Check sheet for the modelled part. Datum: model origin and axes. Units: mm. Face numbers are marked on the shaded views. A direction names the side the tool comes from. Coordinates: 2 decimals unless noted, no trailing zeros. Write each loop counter-clockwise with the first axis right and the second up, starting at its lowest first coordinate (ties: lowest second). Pieces come first, ordered by that corner, then holes. Notation, with made-up numbers: M 21.25,10.25 L 28.25,10.25 A13 ccw 28.25,26.25 Z; hole C -4,-12 d4. An arc over 180 degrees is marked long. Answer as CSV lines item,"result". Start each with the question number.
Q1. Thickness scan on line 1 along Y through (x, z) = (-0.5, -3); line 2 along X through (y, z) = (3.5, -1.5). Record the ranges inside material, lowest first. Write a range as from..to.
Q2. Sectioned sample at C-C, the plane x = 0. Record the cut outline in (y, z), then the cut area to 3 significant figures.
Q3. Mould release check, pull along Y, two halves, no side actions. Record for the marked faces 4, 5 and 6: pulls with the +Y half, pulls with the -Y half, needs draft (parallel to the pull), parting line crosses it, or undercut.
Q4. Sectioned sample at A-A, the plane x = -7. Record the cut outline in (y, z).
Q5. Sectioned sample at D-D, the plane z = 0. Record the cut outline in (x, y), then the cut area to 3 significant figures.
Q6. Depth check by flat-ended pin: pin 1 Ø1.1 at (x, y) = (-8.5, 0.5) entering from +Z; pin 2 Ø5 at (x, y) = (2, 10) entering from +Z; pin 3 Ø2 at (x, y) = (-1, 1) entering from +Z. Enter the tip coordinate at first touch or a pass-through.
Q7. Sectioned sample at B-B, the plane z = 5.5. Record the cut outline in (x, y), then the cut area to 3 significant figures.
Q8. Access from +Z, -Z, +X, -X, +Y, -Y to the whole of each face (thin tool, end or side, straight path). Record for the marked faces 1, 2 and 3.
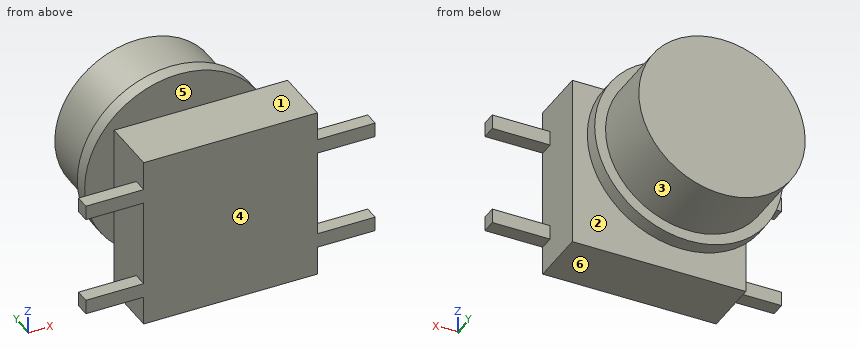
from build123d import *

# Parameters (mm, degrees)
SKETCH1_W               = 12
SKETCH1_H               = 12
BOSS_EXTRUDE1_DEPTH     = 4
SKETCH2_R               = 2.75
BOSS_EXTRUDE2_DEPTH     = 3
SKETCH3_R               = 6.5
BOSS_EXTRUDE3_DEPTH     = 1
BOSS_EXTRUDE4_START     = -1
SKETCH4_R               = 5.75
BOSS_EXTRUDE4_DEPTH     = 5.5
SKETCH5_W               = 1
SKETCH5_H               = 1
BOSS_EXTRUDE5_DEPTH     = 4
MIRROR2_COPY_1_SKETCH_W = 1
MIRROR2_COPY_1_SKETCH_H = 1
MIRROR2_COPY_1_DEPTH    = 4


with BuildPart() as part:
    # Sketch1 → Boss-Extrude1 (new body)
    with BuildSketch(Plane(origin=(0, 0, 0), x_dir=(1, 0, 0), z_dir=(0, 1, 0))):
        Rectangle(SKETCH1_W, SKETCH1_H)
    extrude(amount=BOSS_EXTRUDE1_DEPTH)

    # Sketch2 → Boss-Extrude2 (add)
    with BuildSketch(Plane(origin=(0, 4, 0), x_dir=(1, 0, 0), z_dir=(0, 1, 0))):
        with Locations(Location((0, 0, 0), (0, 0, 270))):
            Circle(SKETCH2_R)
    extrude(amount=BOSS_EXTRUDE2_DEPTH)

    # Sketch3 → Boss-Extrude3 (add)
    with BuildSketch(Plane(origin=(0, 7, 0), x_dir=(1, 0, 0), z_dir=(0, 1, 0))):
        with Locations(Location((0, 0, 0), (0, 0, 270))):
            Circle(SKETCH3_R)
    extrude(amount=BOSS_EXTRUDE3_DEPTH)

    # Sketch4 → Boss-Extrude4 (add)
    with BuildSketch(Plane(origin=(0, 8, 0), x_dir=(1, 0, 0), z_dir=(0, 1, 0)).offset(BOSS_EXTRUDE4_START)):
        with Locations(Location((0, 0, 0), (0, 0, 270))):
            Circle(SKETCH4_R)
    extrude(amount=BOSS_EXTRUDE4_DEPTH)

    # Sketch5 → Boss-Extrude5 (add)
    with BuildSketch(Plane(origin=(6, 0, 0), x_dir=(0, 0, -1), z_dir=(1, 0, 0))):
        with Locations((-3.5, 0.5)):
            Rectangle(SKETCH5_W, SKETCH5_H)
    boss_extrude5 = extrude(amount=BOSS_EXTRUDE5_DEPTH)

    # Mirror1: Boss-Extrude5 across plane
    add(boss_extrude5.mirror(Plane.XY))

    # Mirror2: Boss-Extrude5 across plane
    add(boss_extrude5.mirror(Plane(origin=(0, 0, 0), x_dir=(0, 0, 1), z_dir=(1, 0, 0))))

    # Mirror2 copy 1 sketch → Mirror2 copy 1 (add)
    with BuildSketch(Plane.ZY.offset(6)):
        with Locations((-3.5, 0.5)):
            Rectangle(MIRROR2_COPY_1_SKETCH_W, MIRROR2_COPY_1_SKETCH_H)
    extrude(amount=MIRROR2_COPY_1_DEPTH)


solid = part.part
Output:
1,line 1,"y = 0..4, 7..12.5"
1,line 2,"x = -6..6"
2,outline,"M 0,-6 L 4,-6 L 4,-2.75 L 7,-2.75 L 7,-6.5 L 8,-6.5 L 8,-5.75 L 12.5,-5.75 L 12.5,5.75 L 8,5.75 L 8,6.5 L 7,6.5 L 7,2.75 L 4,2.75 L 4,6 L 0,6 Z"
2,area,"129 mm^2"
3,face 4,"pulls with the -Y half"
3,face 5,"undercut"
3,face 6,"needs draft"
4,outline,"M 0,-4 L 1,-4 L 1,-3 L 0,-3 Z; M 0,3 L 1,3 L 1,4 L 0,4 Z"
5,outline,"M -6.5,7 L -2.75,7 L -2.75,4 L -6,4 L -6,0 L 6,0 L 6,4 L 2.75,4 L 2.75,7 L 6.5,7 L 6.5,8 L 5.75,8 L 5.75,12.5 L -5.75,12.5 L -5.75,8 L -6.5,8 Z"
5,area,"129 mm^2"
6,pin 1,"stops at z = 4"
6,pin 2,"stops at z = 6.48"
6,pin 3,"stops at z = 6"
7,outline,"M -6,0 L 6,0 L 6,4 L -6,4 Z; M -3.46,7 L 3.46,7 L 3.46,8 L 1.68,8 L 1.68,12.5 L -1.68,12.5 L -1.68,8 L -3.46,8 Z"
7,area,"70.0 mm^2"
8,face 1,"+Z, +X, -X, -Y"
8,face 2,"none"
8,face 3,"+Y"
